Can you work these out from the drawing? Everything is in mm from the part's minimum corner. A direction names the side the tool comes from. Round coordinates to 2 decimals unless told otherwise and drop trailing zeros. Loops run counter-clockwise (first coordinate to the right, second up) from the corner with the lowest first, then second, coordinate; pieces in that order, holes last. Notation, with made-up numbers: (-6, 81) -> (18, 81) arc R29 cw to (18, 106) -> close; hole circle Ø4 at (-7, 51). An arc over 180 degrees is marked (long way). One line per item, written item: value.
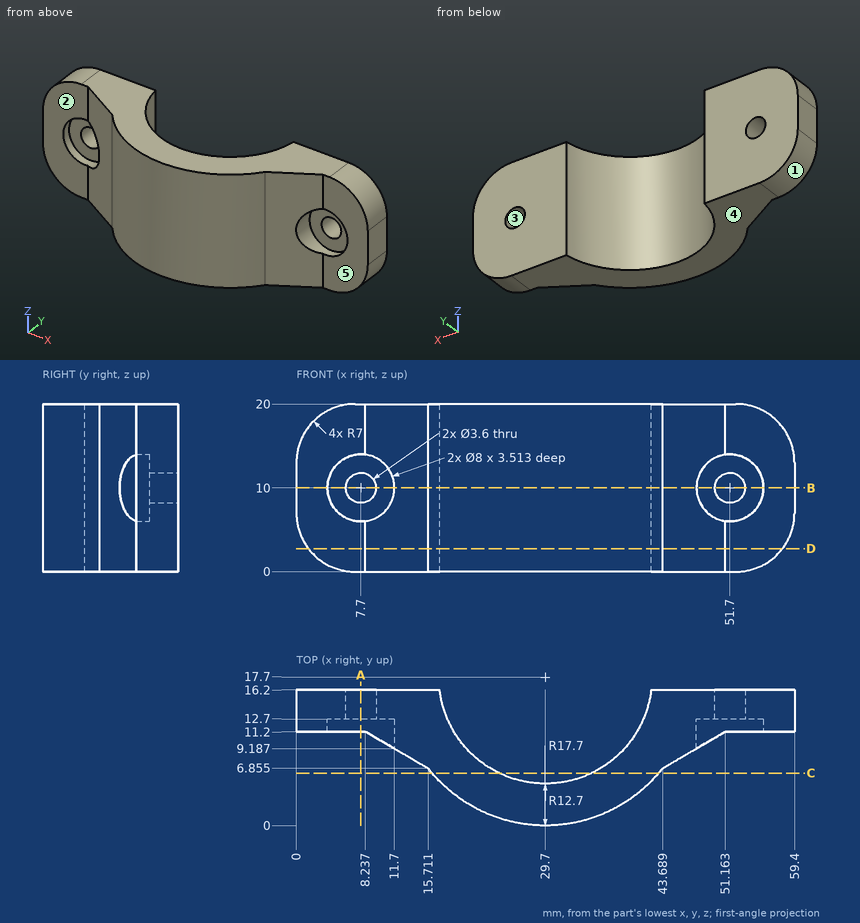
Item 1: For the marked faces 4 and 5, which set-ups out of +Z, -Z, +X, -X, +Y, -Y let a thin tool reach every point of the face, with its end or its side?
Output:
face 4: -Z, +X, -X, +Y, -Y
face 5: +Z, -Z, +X, -Y
Item 2: If we section it at B-B on z = 10: List the corners of the cut face in (x, y) for me (1 decimal).
Output:
outline: (0, 11.2) -> (3.7, 11.2) -> (3.7, 12.7) -> (5.9, 12.7) -> (5.9, 16.2) -> (0, 16.2) -> close; (9.5, 12.7) -> (11.7, 12.7) -> (11.7, 9.2) -> (15.7, 6.9) arc R17.7 ccw to (43.7, 6.9) -> (47.7, 9.2) -> (47.7, 12.7) -> (49.9, 12.7) -> (49.9, 16.2) -> (42.3, 16.2) arc R12.7 cw to (17.1, 16.2) -> (9.5, 16.2) -> close; (53.5, 12.7) -> (55.7, 12.7) -> (55.7, 11.2) -> (59.4, 11.2) -> (59.4, 16.2) -> (53.5, 16.2) -> close
Item 3: I need wall thicknesses on line 1 (Z direction, x = 51.7, y = 14.3); line 2 (X direction, y = 8.75, z = 19); line 3 (Y direction, x = 29.5, z = 17.25). Which ranges of each line are inside material? Lowest first, please. Write a range as from..to.
Output:
line 1: z = 0..8.2, 11.8..20
line 2: x = 12.45..20.69, 38.71..46.95
line 3: y = 0..5
Item 4: If we section it at D-D on z = 2.75: List the corners of the cut face in (x, y) for me (1 decimal), plus the area to 3 significant figures.
Output:
outline: (1.4, 11.2) -> (8.2, 11.2) -> (15.7, 6.9) arc R17.7 ccw to (43.7, 6.9) -> (51.2, 11.2) -> (58, 11.2) -> (58, 16.2) -> (42.3, 16.2) arc R12.7 cw to (17.1, 16.2) -> (1.4, 16.2) -> close
area: 355 mm²
Item 5: Will these pins go through, and if not, where does the flat tip stop? pin 1 Ø10.5 at (x, z) = (51.7, 10) entering from -Y; pin 2 Ø2.5 at (x, z) = (55, 8.5) entering from -Y; pin 3 Ø8 at (x, z) = (43, 9) entering from -Y; pin 4 Ø3 at (x, z) = (51.7, 10) entering from -Y.
Output:
pin 1: stops at y = 8.46
pin 2: stops at y = 11.2
pin 3: stops at y = 2.64
pin 4: passes through
Item 6: If we section it at C-C on y = 6.25: List the corners of the cut face in (x, z) for me, plus the area to 3 significant figures.
Output:
outline: (16.2, 0) -> (24.21, 0) -> (24.21, 20) -> (16.2, 20) -> close; (35.19, 0) -> (43.2, 0) -> (43.2, 20) -> (35.19, 20) -> close
area: 320 mm²
Item 7: If we section it at A-A on x = 7.7: List the corners of the cut face in (y, z) for me.
Output:
outline: (11.2, 0) -> (16.2, 0) -> (16.2, 8.2) -> (12.7, 8.2) -> (12.7, 6) -> (11.2, 6) -> close; (11.2, 14) -> (12.7, 14) -> (12.7, 11.8) -> (16.2, 11.8) -> (16.2, 20) -> (11.2, 20) -> close
Item 8: If we mould it in two halves opening along Z, with no side actions, what happens to the marked faces 1, 2 and 3? For each: released by +Z, released by -Z, zero draft, split by the parting line, or undercut.
Output:
face 1: released by -Z
face 2: zero draft
face 3: undercut
